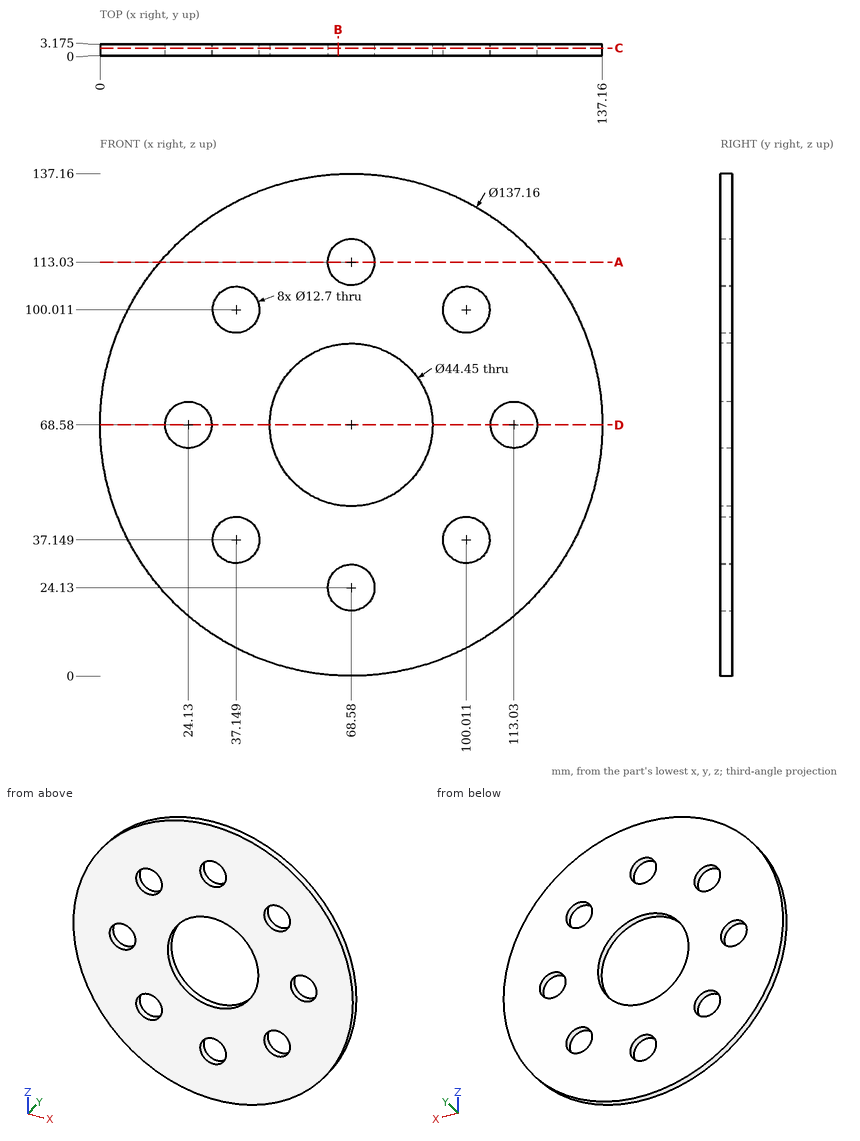
The drawing under review shows one solid part. Ordinate dimensions are in mm from its lowest x, y, z. Give positions to 0.01 mm unless a question says otherwise; leave off trailing zeros. Order: outer loops, then holes, each group sorted by start corner. A loop starts at its lowest first (then second) coordinate and runs counter-clockwise, first axis right, second up. Notation, with made-up numbers: (59.25, 47) -> (89.25, 47) arc R15 ccw to (89.25, 71) -> close; hole circle Ø3 at (79, 25). An arc over 180 degrees is marked (long way). Write item = value, one per line. Start each with the question number.
(1) To check wall thickness, follow line 1 along Z through (x, y) = (68.58, 0.95) (3 decimals); line 2 along Z through (x, y) = (70.5, 2.55). State the ranges of each line that lie inside material, in increasing order.
(2) For pin 1 (4 mm diameter, centred on x = 34.5, z = 76.5, fed in from -Y); pin 2 (1.5 mm diameter, centred on y = 1, z = 29.5, fed in from -X); pin 3 (1.5 mm diameter, centred on x = 39, y = 1, fed in from -Z), all flat-tipped, find the tip position at first contact; note any pin that passes through.
(3) We need section C-C on y = 2.05. State how many separate pieces and enclosed holes the cut face has, plus the area to 3 significant figures.
(4) We need section A-A on z = 113.03. Write out the cut boundary in (x, y) (1 decimal), plus the area to 3 significant figures.
(5) We need section D-D on z = 68.58. Write out the cut boundary in (x, y) (3 decimals).
(6) We need section B-B on x = 65. Write out the cut boundary in (y, z) (1 decimal), plus the area to 3 significant figures.
Numbers:
q1.line_1 = 0 to 17.78, 30.48 to 46.355, 90.805 to 106.68, 119.38 to 137.16
q1.line_2 = 0.03 to 18.08, 30.18 to 46.44, 90.72 to 106.98, 119.08 to 137.13
q2.pin_1 = 0
q2.pin_2 = 11.71
q2.pin_3 = 6.35
q3.separate_pieces = 1
q3.enclosed_holes = 9
q3.area = 12,200 mm^2
q4.outline = (16.4, 0) -> (62.2, 0) -> (62.2, 3.2) -> (16.4, 3.2) -> close; (74.9, 0) -> (120.8, 0) -> (120.8, 3.2) -> (74.9, 3.2) -> close
q4.area = 291 mm^2
q5.outline = (0, 0) -> (17.78, 0) -> (17.78, 3.175) -> (0, 3.175) -> close; (30.48, 0) -> (46.355, 0) -> (46.355, 3.175) -> (30.48, 3.175) -> close; (90.805, 0) -> (106.68, 0) -> (106.68, 3.175) -> (90.805, 3.175) -> close; (119.38, 0) -> (137.16, 0) -> (137.16, 3.175) -> (119.38, 3.175) -> close
q6.outline = (0, 0.1) -> (3.2, 0.1) -> (3.2, 18.9) -> (0, 18.9) -> close; (0, 29.4) -> (3.2, 29.4) -> (3.2, 46.6) -> (0, 46.6) -> close; (0, 90.5) -> (3.2, 90.5) -> (3.2, 107.8) -> (0, 107.8) -> close; (0, 118.3) -> (3.2, 118.3) -> (3.2, 137.1) -> (0, 137.1) -> close
q6.area = 229 mm^2
